The model under review builds one solid part; all positions refer to its coordinate system, in mm. Coordinates: 2 decimals unless noted, no trailing zeros. Order: outer loops, then holes, each group sorted by start corner. A loop starts at its lowest first (then second) coordinate and runs counter-clockwise, first axis right, second up. Notation, with made-up numbers: M 25,-0.75 L 33,-0.75 A9 cw 33,10.25 Z; hole C 42.5,83 d8. An arc over 180 degrees is marked long. Answer as CSV lines item,"result". Start each with the question number.
Q1. For P1, Ø4, axis at x = 12.5, y = 0, coming from the +Z side, flat-tipped, find the tip position at first contact; note if it passes through.
Q2. Consider section A-A on x = 0. Write out the cut boundary in (y, z).
Q3. Wall thickness on L1, parallel to Y at x = -12.5, z = 1.1; L2, parallel to X at y = 9, z = 3.7; L3, parallel to X at y = -8, z = 3.15: over which ranges is each line inside the solid? List them lowest first. Write a range as [from, to].
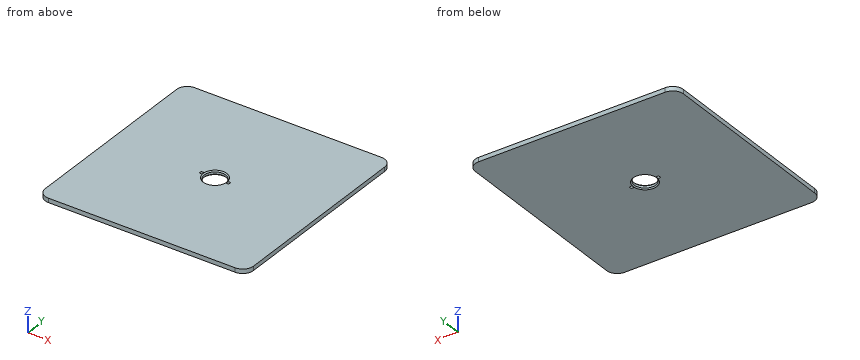
from build123d import *

# Parameters (mm, degrees)
F0_W     = 194
F0_H     = 194
F0_R     = 1.5
F0_R_2   = 10
F1_DEPTH = 4
F2_SIZE  = 0.99999
F3_R     = 10


# Not quite as in the source:
# - a fillet or chamfer is up to 0.001 mm smaller than in the source, because OpenCascade refuses the exact size


with BuildPart() as f1:
    # F0 (on Top) → F1 (new body)
    with BuildSketch(Plane.XY):
        Rectangle(F0_W, F0_H)
        with Locations((-12.5, 0)):
            Circle(F0_R, mode=Mode.SUBTRACT)
        Circle(F0_R_2, mode=Mode.SUBTRACT)
        with Locations((12.5, 0)):
            Circle(F0_R, mode=Mode.SUBTRACT)
    extrude(amount=F1_DEPTH)

    # F2 (size 1 in the source; OpenCascade refuses exactly that, so slightly less here)
    f2_edges = [f1.edges().sort_by_distance(p)[0] for p in [
        (-10, 0, 4),
        (-10, 0, 0),
    ]]
    chamfer(f2_edges, length=F2_SIZE)

    # F3
    f3_edges = [f1.edges().sort_by_distance(p)[0] for p in [
        (-97, 97, 2),
        (-97, -97, 2),
        (97, -97, 2),
        (97, 97, 2),
    ]]
    fillet(f3_edges, radius=F3_R)


solid = f1.part
Evaluation:
1,P1,"stops at z = 4"
2,outline,"M -97,0 L -11,0 L -10,1 L -10,3 L -11,4 L -97,4 Z; M 10,1 L 11,0 L 97,0 L 97,4 L 11,4 L 10,3 Z"
3,L1,"y = [-97, -1.5], [1.5, 97]"
3,L2,"x = [-97, -5.79], [5.79, 97]"
3,L3,"x = [-97, -6.25], [6.25, 97]"
